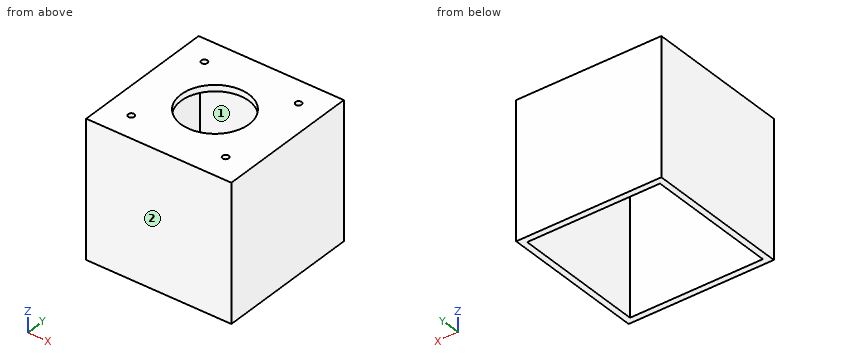
Solid Edge part; units mm, degrees
sketch "Sketch1" plane through (0, 0, 0) normal (0, 0, 1) x (1, 0, 0)
  line L0 (-21.5, 21.5001) -> (-21.5, -21.4999)
  line L1 (-21.5, -21.4999) -> (21.5, -21.4999)
  line L2 (21.5, -21.4999) -> (21.5, 21.5001)
  line L3 (21.5, 21.5001) -> (-21.5, 21.5001)
extrude "Protrusion1" add sketch "Sketch1" against normal blind 42
shell "Thinwall_1" thickness 0 removed faces 1 at (-14.7633, -13.9032, -42) outside thickness 2
hole "Hole_1" at (15.2665, -15.2666, 2) direction (0, 0, -1) diameter 2 end up to next
hole "Hole1" at (-15.2665, -15.2665, 2) direction (0, 0, -1) diameter 2 end up to next
hole "Hole2" at (-15.2665, 15.2665, 2) direction (0, 0, -1) diameter 2 end up to next
hole "Hole3" at (15.2664, 15.2664, 2) direction (0, 0, -1) diameter 2 end up to next
hole "Hole_6" at (-0.0001, 0, 2) direction (0, 0, -1) diameter 22 end up to next
Input: part model. Units: mm. Frame: model coordinates. Face numbers are marked on the shaded views. A direction names the side the tool comes from. Coordinates: 2 decimals unless noted, no trailing zeros. Loops run counter-clockwise (first coordinate to the right, second up) from the corner with the lowest first, then second, coordinate; pieces in that order, holes last.
(1) First-contact query: pin 1 Ø6 at (x, y) = (-2, -14.5) entering from -Z. Flat tip, straight axial feed; report the tip coordinate or a pass-through.
(2) Set-up query: the marked faces 1 and 2. Return all of +Z, -Z, +X, -X, +Y, -Y with unobstructed straight access to the full face (end or side cutting, diameter ignored); none if empty.
(3) Section B-B on z = -15.5. Return the cut outline in (x, y).
(4) Material intervals for probe 1 along Y at (x, z) = (-7, -28); probe 2 along X at (y, z) = (0, 1.5), sorted ascending.
(5) Section A-A on y = 0. Return the cut outline in (x, z).
(6) Section C-C on y = 18. Return the cut outline in (x, z), then the cut area to 3 significant figures.
Data:
1. pin 1: stops at z = 0
2. face 1: -Z
2. face 2: +Z, -Z, +X, -X, -Y
3. outline: (-23.5, -23.5) - (23.5, -23.5) - (23.5, 23.5) - (-23.5, 23.5) - close; hole (-21.5, -21.5) - (21.5, -21.5) - (21.5, 21.5) - (-21.5, 21.5) - close
4. probe 1: y = -23.5 to -21.5, 21.5 to 23.5
4. probe 2: x = -23.5 to -11, 11 to 23.5
5. outline: (-23.5, -42) - (-21.5, -42) - (-21.5, 0) - (-11, 0) - (-11, 2) - (-23.5, 2) - close; (11, 0) - (21.5, 0) - (21.5, -42) - (23.5, -42) - (23.5, 2) - (11, 2) - close
6. outline: (-23.5, -42) - (-21.5, -42) - (-21.5, 0) - (21.5, 0) - (21.5, -42) - (23.5, -42) - (23.5, 2) - (-23.5, 2) - close
6. area: 262 mm2
